Can you work these out from the model? Positions are in its coordinate system, mm. Face numbers are marked on the shaded views. A direction names the side the tool comes from. Round coordinates to 2 decimals unless told otherwise and drop trailing zeros. Write each loop counter-clockwise with the first axis right and the second up, starting at its lowest first coordinate (ties: lowest second). Pieces come first, ordered by that corner, then holes.
Q1. If we section it at B-B (y = -4.75): Please give me the cut outline in (x, z).
Q2. If we section it at A-A (z = -30): Please give me the cut outline in (x, y).
Q3. If we section it at C-C (x = -10): Please give me the cut outline in (y, z).
Q4. We'd pull the mould along Z, two halves only. Please class the marked faces 1 and 2: +Z half, -Z half, draft (parallel to the pull), parting line (faces both ways), or undercut.
Q5. For the marked faces 3 and 4, which set-ups out of +Z, -Z, +X, -X, +Y, -Y let a thin tool reach every point of the face, with its end or its side?
Q6. If we section it at D-D (z = 27): Please give me the cut outline in (x, y).
Q7. I'm going to push a flat-ended pin straight in: pin 1 Ø12 at (x, z) = (-9.5, 29.5) entering from -Y. Where does the tip first touch, or does it pass through?
Q8. Please list where these lines run through material, in increasing order: line 1 along Z through (x, y) = (6, -2.25); line 2 along X through (y, z) = (-4.75, 37); line 3 along Y through (x, z) = (-0.5, 42.5).
Autodesk Inventor part; units mm, degrees
ref_plane "YZ Plane" through (0, 0, 0) normal (1, 0, 0) x (0, 1, 0)
ref_plane "XZ Plane" through (0, 0, 0) normal (0, 1, 0) x (-1, 0, 0)
ref_plane "XY Plane" through (0, 0, 0) normal (0, 0, 1) x (1, 0, 0)
sketch "Boceto1" plane through (0, 0, 0) normal (0, 1, 0) x (-1, 0, 0)
  line L0 (20.25, -43.5) -> (-20.25, -43.5)
  line L1 (-20.25, -43.5) -> (-20.25, 43.5)
  line L2 (-20.25, 43.5) -> (20.25, 43.5)
  line L3 (20.25, 43.5) -> (20.25, -43.5)
  line L4 (20.25, -43.5) -> (-20.25, 43.5) construction
  line L5 (-20.25, -43.5) -> (20.25, 43.5) construction
  line L6 (25.25, -48.5) -> (-25.25, -48.5)
  line L7 (-25.25, -48.5) -> (-25.25, 48.5)
  line L8 (-25.25, 48.5) -> (25.25, 48.5)
  line L9 (25.25, 48.5) -> (25.25, -48.5)
  line L10 (20.25, 43.5) -> (-20.25, 43.5)
  line L11 (-20.25, 43.5) -> (-20.25, 14)
  line L12 (-20.25, 14) -> (20.25, 14)
  line L13 (20.25, 14) -> (20.25, 43.5)
  line L14 (25.25, 14) -> (-25.25, 14)
  line L15 (21.25, -44.5) -> (-21.25, -44.5)
  line L16 (-21.25, -44.5) -> (-21.25, 44.5)
  line L17 (-21.25, 44.5) -> (21.25, 44.5)
  line L18 (21.25, 44.5) -> (21.25, -44.5)
  line L19 (8.5, 14) -> (-8.5, 14)
  line L20 (-8.5, 14) -> (-8.5, 16)
  line L21 (-8.5, 16) -> (8.5, 16)
  line L22 (8.5, 16) -> (8.5, 14)
  point P0 (0, 0)
  point P1 (0, 0)
  point P2 (-20.25, 14)
  point P3 (20.25, 14)
  point P4 (-20.25, 14)
  point P5 (0, 14)
  point P6 (-8.5, 14)
  dimension "d0" = 40.5
  dimension "d1" = 87
  dimension "d2" = 5
  dimension "d3" = 29.5
  dimension "d19" = 1
  dimension "d20" = 17
  dimension "d21" = 2
extrude "Extrusión4" add sketch "Boceto1" against normal blind 7.5 contours L3 L14 L18 L15 L16 L1 L0 | L3 L2 L1 L14 L16 L17 L18 | L18 L17 L16 L14 L7 L8 L9 | L14 L9 L6 L7 L16 L15 L18
extrude "Extrusión5" add sketch "Boceto1" along normal blind 1 contours L3 L14 L18 L15 L16 L1 L0 | L12 L22 L21 L20 L1 L2 L3 | L3 L2 L1 L14 L16 L17 L18 | L18 L17 L16 L14 L7 L8 L9 | L14 L9 L6 L7 L16 L15 L18
fillet "Empalme2" radius 4 4 edges at (-20.25, -3.25, -43.5) (20.25, -3.25, -43.5) (20.25, -3.75, 43.5) (-20.25, -3.75, 43.5)
fillet "Empalme3" radius 2 2 edges at (14.375, 0, 14) (-14.375, 0, 14)
properties part number "manija_puerta_marco_front_right_v2"
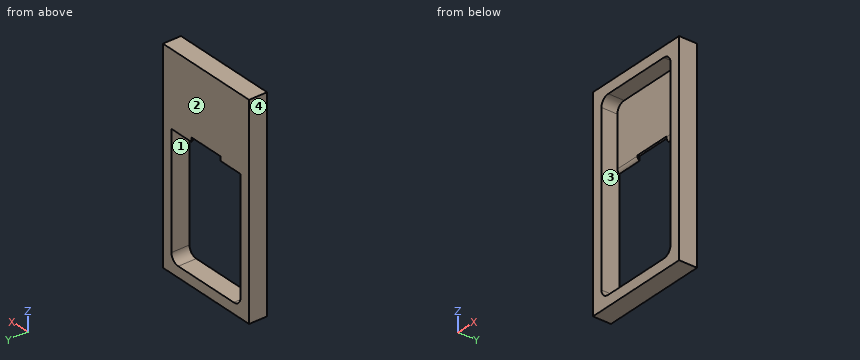
A:
1. outline: (-25.25, -48.5) - (25.25, -48.5) - (25.25, 48.5) - (-25.25, 48.5) - close; hole (-20.25, -39.5) arc R4 ccw to (-16.25, -43.5) - (16.25, -43.5) arc R4 ccw to (20.25, -39.5) - (20.25, 39.5) arc R4 ccw to (16.25, 43.5) - (-16.25, 43.5) arc R4 ccw to (-20.25, 39.5) - close
2. outline: (-25.25, -7.5) - (-20.25, -7.5) - (-20.25, 1) - (-25.25, 1) - close; (20.25, -7.5) - (25.25, -7.5) - (25.25, 1) - (20.25, 1) - close
3. outline: (-7.5, -48.5) - (1, -48.5) - (1, -43.5) - (-7.5, -43.5) - close; (-7.5, 43.5) - (0, 43.5) - (0, 15.73) arc R2 ccw to (1, 14) - (1, 48.5) - (-7.5, 48.5) - close
4. face 1: undercut
4. face 2: draft
5. face 3: -Y
5. face 4: +Z, -Z, -X, +Y, -Y
6. outline: (-25.25, -7.5) - (-20.25, -7.5) - (-20.25, 0) - (20.25, 0) - (20.25, -7.5) - (25.25, -7.5) - (25.25, 1) - (-25.25, 1) - close
7. pin 1: stops at y = 0
8. line 1: z = -48.5 to -43.5, 43.5 to 48.5
8. line 2: x = -25.25 to -20.25, 20.25 to 25.25
8. line 3: y = 0 to 1
